Here's how the part is built. I have some questions about the finished solid (model axes, mm). Round coordinates to 2 decimals unless told otherwise and drop trailing zeros. Write each loop counter-clockwise with the first axis right and the second up, starting at its lowest first coordinate (ties: lowest second). Pieces come first, ordered by that corner, then holes. Notation, with made-up numbers: (19, 58.25) -> (47, 58.25) arc R14 cw to (47, 72.25) -> close; hole circle Ø5 at (2.5, 36). An arc over 180 degrees is marked (long way). Answer in a Markdown table with one row per item.
Autodesk Inventor part; units mm, degrees
ref_plane "YZ Plane" through (0, 0, 0) normal (1, 0, 0) x (0, 1, 0)
ref_plane "XZ Plane" through (0, 0, 0) normal (0, 1, 0) x (-1, 0, 0)
ref_plane "XY Plane" through (0, 0, 0) normal (0, 0, 1) x (1, 0, 0)
sketch "Sketch1" plane through (0, 0, 0) normal (0, 1, 0) x (-1, 0, 0)
  line L0 (0, 0) -> (-38.1, 0)
  line L1 (-38.1, 0) -> (-38.1, -38.1)
  line L2 (-38.1, -38.1) -> (0, -38.1)
  line L3 (0, -38.1) -> (0, 0)
  line L4 (-3.175, -3.175) -> (-34.925, -3.175)
  line L5 (-34.925, -3.175) -> (-34.925, -34.925)
  line L6 (-34.925, -34.925) -> (-3.175, -34.925)
  line L7 (-3.175, -34.925) -> (-3.175, -3.175)
  dimension "d0" = 38.1
  dimension "d1" = 38.1
  dimension "d2" = 3.175
extrude "Extrusion1" add sketch "Sketch1" along normal blind 809.625
sketch "Sketch2" plane through (38.1, 0, 0) normal (1, 0, 0) x (0, 0, -1)
  circle A0 centre (19.05, 784.225) radius 6.35
  line L0 (0, 809.625) -> (38.1, 809.625)
  point P0 (0, 0)
  dimension "d5" = 12.7
  dimension "d6" = 25.4
extrude "Extrusion2" cut sketch "Sketch2" against normal through all
properties part number "Pivot point Support"
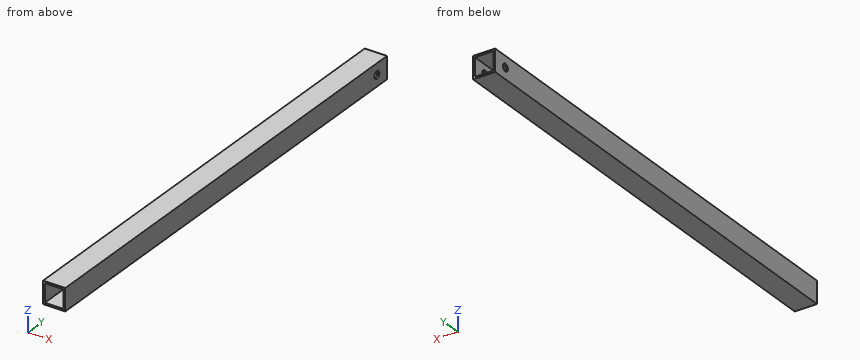
1) I want a section at A-A, the plane z = -19.05. List the corners of the cut face in (x, y) for me (3 decimals).
Response:
| item | result |
|---|---|
| outline | (0, 0) -> (3.175, 0) -> (3.175, 777.875) -> (0, 777.875) -> close; (0, 790.575) -> (3.175, 790.575) -> (3.175, 809.625) -> (0, 809.625) -> close; (34.925, 0) -> (38.1, 0) -> (38.1, 777.875) -> (34.925, 777.875) -> close; (34.925, 790.575) -> (38.1, 790.575) -> (38.1, 809.625) -> (34.925, 809.625) -> close |
2) I want a section at C-C, the plane y = 679. List the corners of the cut face in (x, z) for me (3 decimals).
Response:
| item | result |
|---|---|
| outline | (0, -38.1) -> (38.1, -38.1) -> (38.1, 0) -> (0, 0) -> close; hole (3.175, -34.925) -> (34.925, -34.925) -> (34.925, -3.175) -> (3.175, -3.175) -> close |
3) I want a section at B-B, the plane x = 11.5. List the corners of the cut face in (y, z) for me (3 decimals).
Response:
| item | result |
|---|---|
| outline | (0, -38.1) -> (809.625, -38.1) -> (809.625, -34.925) -> (0, -34.925) -> close; (0, -3.175) -> (809.625, -3.175) -> (809.625, 0) -> (0, 0) -> close |
4) I need wall thicknesses on line 1 (X direction, y = 279, z = -15) (3 decimals); line 2 (Y direction, x = 36.25, z = -19.05) (3 decimals); line 3 (Z direction, x = 8.5, y = 235) (3 decimals). Which ranges of each line are inside material? Lowest first, please. Write a range as [from, to].
Response:
| item | result |
|---|---|
| line 1 | x = [0, 3.175], [34.925, 38.1] |
| line 2 | y = [0, 777.875], [790.575, 809.625] |
| line 3 | z = [-38.1, -34.925], [-3.175, 0] |
5) For pin 1 (9.5 mm diameter, centred on y = 545.5, z = -14.5, fed in from -X); pin 2 (10 mm diameter, centred on y = 784.225, z = -19.05, fed in from -X), each with a flat end and sliding along its axis, tell me the tip position at first contact or that it passes through.
Response:
| item | result |
|---|---|
| pin 1 | stops at x = 0 |
| pin 2 | passes through |
